```python
from build123d import *

# Parameters (mm, degrees)
CHAMFER1_SIZE       = 1
SKETCH2_R           = 54
BOSS_EXTRUDE1_DEPTH = 15.858462


with BuildPart() as part:
    # Sketch1 → Revolve3 (revolve)
    with BuildSketch(Plane(origin=(0, 0, 0), x_dir=(0, 0, -1), z_dir=(1, 0, 0))):
        with BuildLine():
            Line((-458.414283312, 54), (-458.414283312, 63.3349))
            Line((-458.414283312, 63.3349), (-442.555821638, 63.3349))
            Line((-442.555821638, 63.3349), (-442.555821638, 54))
            ThreePointArc((-442.555821638, 54), (-443.54515622, 27.008055426), (-443.875, 0))
            Line((-443.875, 0), (-451.375, 0))
            ThreePointArc((-451.375, 0), (-453.142234121, 27.228438761), (-458.414283312, 54))
        make_face()
    revolve(axis=Axis((0, 0, 662.018), (0, 0, -1)))

    # Chamfer1
    chamfer1_edges = [part.edges().sort_by_distance(p)[0] for p in [
        (0, -63.3349, 442.555821638),
        (0, -63.3349, 458.414283312),
    ]]
    chamfer(chamfer1_edges, length=CHAMFER1_SIZE)

    # Sketch2 → Boss-Extrude1 (add)
    with BuildSketch(Plane.XY.offset(458.414283312)):
        Circle(SKETCH2_R)
    extrude(amount=-BOSS_EXTRUDE1_DEPTH)


solid = part.part
```
Can you work these out from the model? Positions are in its coordinate system, mm. Coordinates: 2 decimals unless noted, no trailing zeros. Loops run counter-clockwise (first coordinate to the right, second up) from the corner with the lowest first, then second, coordinate; pieces in that order, holes last.
1) Imagine slicing it at A-A on z = 450.25. List the corners of the cut face in (x, y) for me, plus the area to 3 significant figures.
2) For pin 1 (5 mm diameter, centred on y = -41.5, z = 449, fed in from +X); pin 2 (4 mm diameter, centred on y = -16, z = 453, fed in from -X); pin 3 (1.5 mm diameter, centred on x = 21, z = 452, fed in from +Y), each with a flat end and sliding along its axis, tell me the tip position at first contact or that it passes through.
3) I need wall thicknesses on probe 1 along Y at (x, z) = (11, 448.25); probe 2 along Y at (x, z) = (-1.5, 446.5); probe 3 along X at (y, z) = (-18, 446.5). Which ranges of each line are inside material? Lowest first, please.
Completed:
1. outline: circle Ø126.67 at (0, 0)
1. area: 12,600 mm2
2. pin 1: stops at x = 49.9
2. pin 2: stops at x = -61.77
2. pin 3: stops at y = 60.01
3. probe 1: y = -62.37 to 62.37
3. probe 2: y = -63.32 to 63.32
3. probe 3: x = -60.72 to 60.72
